Check sheet for the modelled part. Datum: model origin and axes. Units: mm. A direction names the side the tool comes from. Coordinates: 2 decimals unless noted, no trailing zeros. Order: outer loops, then holes, each group sorted by start corner. A loop starts at its lowest first (then second) coordinate and runs counter-clockwise, first axis right, second up.
from build123d import *

# Parameters (mm, degrees)
F0_W     = 76.2
F0_H     = 114.3
F0_R     = 2.54
F1_DEPTH = 12.7
F2_R     = 5.08
F4_DEPTH = 6.35
F5_W     = 60.96
F5_H     = 63.5
F6_DEPTH = 19.05
F7_R     = 5.08


with BuildPart() as f1:
    # F0 (on Top) → F1 (new body, symmetric)
    with BuildSketch(Plane.XY):
        Rectangle(F0_W, F0_H)
        with Locations((33.02, 13.97)):
            Circle(F0_R, mode=Mode.SUBTRACT)
    extrude(amount=F1_DEPTH, both=True)

    # F2
    f2_edges = [f1.edges().sort_by_distance(p)[0] for p in [
        (-38.1, -57.15, 0),
        (38.1, -57.15, 0),
        (-38.1, 57.15, 0),
        (38.1, 57.15, 0),
    ]]
    fillet(f2_edges, radius=F2_R)

    # F3 (on face) → F4 (join)
    with BuildSketch(Plane.XY.offset(12.7)):
        with BuildLine():
            Line((-33.02, 57.15), (-38.1, 57.15))
            Line((-38.1, 57.15), (-38.1, 52.07))
            ThreePointArc((-38.1, 52.07), (-36.6121024484, 55.6621024484), (-33.02, 57.15))
        make_face()
        with BuildLine():
            Line((33.02, 57.15), (-33.02, 57.15))
            ThreePointArc((-33.02, 57.15), (-36.6121024484, 55.6621024484), (-38.1, 52.07))
            Line((-38.1, 52.07), (-38.1, 20.32))
            Line((-38.1, 20.32), (38.1, 20.32))
            Line((38.1, 20.32), (38.1, 52.07))
            ThreePointArc((38.1, 52.07), (36.6121024484, 55.6621024484), (33.02, 57.15))
        make_face()
        with BuildLine():
            Line((38.1, 57.15), (33.02, 57.15))
            ThreePointArc((33.02, 57.15), (36.6121024484, 55.6621024484), (38.1, 52.07))
            Line((38.1, 52.07), (38.1, 57.15))
        make_face()
    extrude(amount=F4_DEPTH)

    # F5 (on face) → F6 (cut)
    with BuildSketch(Plane.XY.offset(12.7)):
        with Locations((-2.54, -19.05)):
            Rectangle(F5_W, F5_H)
    extrude(amount=-F6_DEPTH, mode=Mode.SUBTRACT)

    # F7
    f7_edges = [f1.edges().sort_by_distance(p)[0] for p in [
        (-33.02, 12.7, 3.175),
        (-33.02, -50.8, 3.175),
        (27.94, 12.7, 3.175),
        (27.94, -50.8, 3.175),
        (-38.1, 57.15, 15.875),
        (38.1, 57.15, 15.875),
    ]]
    fillet(f7_edges, radius=F7_R)


solid = f1.part
(1) Cross-section at B-B (x = 16). Enter the section's corners in (y, z), and give its area (3 significant figures).
Filled in:
outline: (-57.15, -12.7) - (57.15, -12.7) - (57.15, 19.05) - (20.32, 19.05) - (20.32, 12.7) - (12.7, 12.7) - (12.7, -6.35) - (-50.8, -6.35) - (-50.8, 12.7) - (-57.15, 12.7) - close
area: 1,930 mm2
(2) Cross-section at A-A (y = 13.97). Enter the section's corners in (x, z).
Filled in:
outline: (-38.1, -12.7) - (30.48, -12.7) - (30.48, 12.7) - (-38.1, 12.7) - close; (35.56, -12.7) - (38.1, -12.7) - (38.1, 12.7) - (35.56, 12.7) - close
(3) Thickness scan on probe 1 along Y at (x, z) = (33.02, -3.5); probe 2 along Y at (x, z) = (-0.5, 9.5); probe 3 along X at (y, z) = (-22, 1). Record the ranges inside material, lowest first.
Filled in:
probe 1: y = -57.15 to 11.43, 16.51 to 57.15
probe 2: y = -57.15 to -50.8, 12.7 to 57.15
probe 3: x = -38.1 to -33.02, 27.94 to 38.1
(4) Tool access check on faces 1 (the flat face through (27.94, -19, 3)), 2 (the flat face through (-1, 20.32, 16)), 3 (the cylindrical face through (36.651, -55.622, 0.178)). Record the directions out of +Z, -Z, +X, -X, +Y, -Y that give a thin tool (end or side, any length) a straight path to the whole face; none if there is none.
Filled in:
face 1: +Z
face 2: +Z, +X, -X, -Y
face 3: +Z, -Z, +X, -Y
(5) Cross-section at D-D (z = 14). Enter the section's corners in (x, y).
Filled in:
outline: (-38.1, 20.32) - (38.1, 20.32) - (38.1, 52.07) arc R5.08 ccw to (33.02, 57.15) - (-33.02, 57.15) arc R5.08 ccw to (-38.1, 52.07) - close
(6) Cross-section at C-C (z = 6). Enter the section's corners in (x, y).
Filled in:
outline: (-38.1, -52.07) arc R5.08 ccw to (-33.02, -57.15) - (33.02, -57.15) arc R5.08 ccw to (38.1, -52.07) - (38.1, 52.07) arc R5.08 ccw to (33.02, 57.15) - (-33.02, 57.15) arc R5.08 ccw to (-38.1, 52.07) - close; hole (-33.02, -45.72) arc R5.08 ccw to (-27.94, -50.8) - (22.86, -50.8) arc R5.08 ccw to (27.94, -45.72) - (27.94, 7.62) arc R5.08 ccw to (22.86, 12.7) - (-27.94, 12.7) arc R5.08 ccw to (-33.02, 7.62) - close; hole circle Ø5.08 at (33.02, 13.97)
(7) Go/stop test with flat-tipped pins: P1, Ø4, axis at x = -17.5, y = -8, coming from the +Z side; P2, Ø4.5, axis at x = 33.02, y = 13.97, coming from the -Z side; P3, Ø3, axis at x = 12, z = 14.5, coming from the -Y side. Record where each tip stops, or that it passes through.
Filled in:
P1: stops at z = -6.35
P2: passes through
P3: stops at y = 20.32
